```python
from build123d import *

# Parameters (mm, degrees)
SKETCH_W    = 80
SKETCH_H    = 88
SKETCH_R    = 11
SKETCH_R_2  = 3
PAD_DEPTH   = 10
FILLET_R    = 10
FILLET001_R = 1


with BuildPart() as part:
    # Sketch → Pad (new body)
    with BuildSketch(Plane.XY):
        with Locations((15, -15)):
            Rectangle(SKETCH_W, SKETCH_H)
        with Locations((0, -30)):
            Circle(SKETCH_R, mode=Mode.SUBTRACT)
        with Locations((-10, -52)):
            Circle(SKETCH_R_2, mode=Mode.SUBTRACT)
        with Locations((40, -52)):
            Circle(SKETCH_R_2, mode=Mode.SUBTRACT)
        with Locations((40, 22)):
            Circle(SKETCH_R_2, mode=Mode.SUBTRACT)
        with Locations((-10, 22)):
            Circle(SKETCH_R_2, mode=Mode.SUBTRACT)
        with BuildLine():
            ThreePointArc((-5, -6.244998), (8, 0), (-5, 6.244998))
            Line((-5, 9), (-5, 6.244998))
            Line((-8.125, 9), (-5, 9))
            Line((-8.125, -9), (-8.125, 9))
            Line((-5, -9), (-8.125, -9))
            Line((-5, -6.244998), (-5, -9))
        make_face(mode=Mode.SUBTRACT)
    extrude(amount=PAD_DEPTH)

    # Fillet
    fillet_edges = [part.edges().sort_by_distance(p)[0] for p in [
        (-25, 29, 5),
        (-25, -59, 5),
    ]]
    fillet(fillet_edges, radius=FILLET_R)

    # Fillet001
    fillet001_edges = [part.edges().sort_by_distance(p)[0] for p in [
        (55, -59, 5),
        (55, 29, 5),
    ]]
    fillet(fillet001_edges, radius=FILLET001_R)


solid = part.part
```
Check sheet for the modelled part. Datum: model origin and axes. Units: mm. A direction names the side the tool comes from. Give positions to 0.01 mm unless a question says otherwise; leave off trailing zeros. Loops run counter-clockwise (first coordinate to the right, second up) from the corner with the lowest first, then second, coordinate; pieces in that order, holes last. Notation, with made-up numbers: M 80.25,-38 L 117.25,-38 A31 ccw 117.25,-4 Z; hole C 76,56 d4. An arc over 180 degrees is marked long. Answer in a Markdown table with one row per item.
1) Cross-section at C-C (y = -30). Enter the section's corners in (x, z).
Solutions:
| item | result |
|---|---|
| outline | M -25,0 L -11,0 L -11,10 L -25,10 Z; M 11,0 L 55,0 L 55,10 L 11,10 Z |
2) Tool access check on faces 1 (the face through (-5, 8, 5)), 2 (the face through (14, -14, 0)). Record the directions out of +Z, -Z, +X, -X, +Y, -Y that give a thin tool (end or side, any length) a straight path to the whole face; none if there is none.
Solutions:
| item | result |
|---|---|
| face 1 | +Z, -Z |
| face 2 | -Z, +X, -X, +Y, -Y |
3) Cross-section at B-B (z = 3). Enter the section's corners in (x, y) (3 decimals).
Solutions:
| item | result |
|---|---|
| outline | M -25,-49 A10 ccw -15,-59 L 54,-59 A1 ccw 55,-58 L 55,28 A1 ccw 54,29 L -15,29 A10 ccw -25,19 Z; hole C -10,-52 d6; hole C -10,22 d6; hole C 0,-30 d22; hole M -8.125,-9 L -5,-9 L -5,-6.245 A8 ccw long -5,6.245 L -5,9 L -8.125,9 Z; hole C 40,-52 d6; hole C 40,22 d6 |
4) Cross-section at D-D (x = -10). Enter the section's corners in (y, z), plus the area to 3 significant figures.
Solutions:
| item | result |
|---|---|
| outline | M -59,0 L -55,0 L -55,10 L -59,10 Z; M -49,0 L -34.58,0 L -34.58,10 L -49,10 Z; M -25.42,0 L 19,0 L 19,10 L -25.42,10 Z; M 25,0 L 29,0 L 29,10 L 25,10 Z |
| area | 668 mm^2 |
5) Mould release check, pull along Y, two halves, no side actions. Record for faces 3 (the face through (55, -16, 5)), 4 (the face through (-8.125, 0, 5)), 5 (the face through (-22.15, -55.99, 5.07)): released by +Y, released by -Y, zero draft, split by the parting line, or undercut.
Solutions:
| item | result |
|---|---|
| face 3 | zero draft |
| face 4 | undercut |
| face 5 | released by -Y |
6) Depth check by flat-ended pin: pin 1 (7 mm diameter, centred on x = -10, y = -52, fed in from -Z); pin 2 (1.5 mm diameter, centred on x = -16, z = 6.5, fed in from -Y); pin 3 (20 mm diameter, centred on x = 0, y = -30, fed in from -Z). Enter the tip coordinate at first touch or a pass-through.
Solutions:
| item | result |
|---|---|
| pin 1 | stops at z = 0 |
| pin 2 | stops at y = -59 |
| pin 3 | passes through |
7) Cross-section at A-A (x = 0). Enter the section's corners in (y, z), plus the area to 3 significant figures.
Solutions:
| item | result |
|---|---|
| outline | M -59,0 L -41,0 L -41,10 L -59,10 Z; M -19,0 L -8,0 L -8,10 L -19,10 Z; M 8,0 L 29,0 L 29,10 L 8,10 Z |
| area | 500 mm^2 |
8) Thickness scan on line 1 (Y direction, x = 40, z = 5); line 2 (Y direction, x = 0, z = 8); line 3 (Y direction, x = -10, z = 6.5). Record the ranges inside material, lowest first.
Solutions:
| item | result |
|---|---|
| line 1 | y = -59 to -55, -49 to 19, 25 to 29 |
| line 2 | y = -59 to -41, -19 to -8, 8 to 29 |
| line 3 | y = -59 to -55, -49 to -34.58, -25.42 to 19, 25 to 29 |
